Could you check a few things on this model? Use its own coordinates, in mm. A direction names the side the tool comes from. Give positions to 0.01 mm unless a question says otherwise; leave off trailing zeros. Write each loop counter-clockwise with the first axis right and the second up, starting at its lowest first coordinate (ties: lowest second). Pieces come first, ordered by that corner, then holes. Notation, with made-up numbers: (11, 27.25) - (30, 27.25) arc R31 ccw to (30, 52.25) - close; hole circle Ø1 at (-38.75, 41.5). An arc over 180 degrees is marked (long way). Use one line per item in the form item = value.
Autodesk Fusion 360 part; units mm, degrees
sketch "草图1" plane through (0, 0, 0) normal (0, 0, 1) x (1, 0, 0) in component "Component"
  line L0 (1.875, 3.2476) -> (3.75, 0)
  line L1 (-1.875, 3.2476) -> (1.875, 3.2476)
  line L2 (-3.75, 0) -> (-1.875, 3.2476)
  line L3 (-1.875, -3.2476) -> (-3.75, 0)
  line L4 (1.875, -3.2476) -> (-1.875, -3.2476)
  line L5 (3.75, 0) -> (1.875, -3.2476)
extrude "拉伸1" add sketch "草图1" along normal blind 3 in component "Component"
sketch "草图2" plane through (0, 0, 0) normal (0, 0, 1) x (1, 0, 0) in component "Component"
  circle A0 centre (0, 0) radius 2.5
extrude "拉伸2" add sketch "草图2" along normal blind 15 in component "Component"
chamfer "倒角1" distance 0.5 angle 45 1 edges at (-2.3308, -0.904, 15) in component "Component"
fillet "圆角1" radius 0.3 1 edges at (-2.3308, 0.904, 3) in component "Component"
sketch "草图3" plane through (0, 0, 0) normal (0, 1, 0) x (1, 0, 0) in component "Component"
  line L0 (3.2476, 0) -> (3.75, 0)
  line L1 (3.75, 0) -> (3.75, -0.1829)
  line L2 (3.75, -0.1829) -> (3.2476, 0)
  line L3 (3.2476, -3) -> (3.75, -3)
  line L4 (3.75, -3) -> (3.75, -2.8171)
  line L5 (3.75, -2.8171) -> (3.2476, -3)
revolve "旋转1" cut sketch "草图3" angle 360 about axis through (0, 0, 1.75) along (0, 0, 1) contours L3 L4 L5 in component "Component"
revolve "旋转2" cut sketch "草图3" angle 360 about axis through (0, 0, 1.75) along (0, 0, 1) contours L0 L1 L2 in component "Component"
thread "螺纹1" in component "Component"
component "Component" placed x (1, 0, 0) y (0, 1, 0) z (0, 0, 1) at (0, 0, 0)
1. For pin 1 (2 mm diameter, centred on y = -2, z = 2.5, fed in from +X); pin 2 (2 mm diameter, centred on y = -1.5, z = 8.5, fed in from -X), each with a flat end and sliding along its axis, tell me the tip position at first contact or that it passes through.
Response values:
pin_1 = 3.17
pin_2 = -2.45
2. Imagine slicing it at B-B, the plane z = 1. List the corners of the cut face in (x, y) for me (3 decimals), and give its area (3 significant figures).
Response values:
outline = (-3.75, 0) - (-1.875, -3.248) - (1.875, -3.248) - (3.75, 0) - (1.875, 3.248) - (-1.875, 3.248) - close
area = 36.5 mm²
3. Imagine slicing it at A-A, the plane z = 6. List the corners of the cut face in (x, y) for me, and give its area (3 significant figures).
Response values:
outline = circle Ø5 at (0, 0)
area = 19.6 mm²
4. If I drill on line 1 (X direction, y = 1.5, z = 10); line 2 (X direction, y = -1.75, z = 2.25); line 3 (Z direction, x = 2.25, y = 0), over which ranges is the centre line in solid material (lowest first)? Write a range as from..to.
Response values:
line_1 = -2..2
line_2 = -2.74..2.74
line_3 = 0..14.75
5. If we mould it in two halves opening along Y, with no side actions, what happens to faces 1 (the face through (-3.426, 0.008, 0.065)), 2 (the face through (-1.72, 2.962, 2.935)), 3 (the face through (-2.799, -1.647, 1.479)), 4 (the face through (0, 0, 15))? For each: pulls with the +Y half, pulls with the -Y half, needs draft (parallel to the pull), parting line crosses it, or undercut.
Response values:
face_1 = parting line crosses it
face_2 = pulls with the +Y half
face_3 = pulls with the -Y half
face_4 = needs draft
6. Which directions (+Z, -Z, +X, -X, +Y, -Y) give clear straight access to the entire face, cutting with the end or side of a thin tool? Please do faces 5 (the face through (0, 3, 3)), 6 (the face through (2.826, -1.601, 1.479)).
Response values:
face_5 = +Z
face_6 = +Z, -Z, +X, -Y
